Verification items for the finished model (mm, model axes). A direction names the side the tool comes from. Coordinates: 2 decimals unless noted, no trailing zeros. Order: outer loops, then holes, each group sorted by start corner. A loop starts at its lowest first (then second) coordinate and runs counter-clockwise, first axis right, second up. Notation, with made-up numbers: M 55.5,45 L 87.5,45 A28 cw 87.5,75 Z; hole C 50,45.25 d2. An arc over 180 degrees is marked long. Return JSON: item names as keys, results as strings. Group by question number.
1. Section check D-D, the plane z = -8. Record the cut outline in (x, y).
2. Set-up check for faces 1 (the flat face through (12, 1, 10)), 2 (the cylindrical face through (15.99, 1.12, 6.58)), 3 (the flat face through (12, 11, 10)), 4 (the flat face through (-12, 6, 0)): record each of +Z, -Z, +X, -X, +Y, -Y from which the full face is reachable in a straight line by a thin tool's end or side.
3. Section check A-A, the plane z = 9.5. Record the cut outline in (x, y).
4. Section check B-B, the plane y = 2. Record the cut outline in (x, z).
5. Material ranges on line 1 along X through (y, z) = (10.25, -2.25); line 2 along X through (y, z) = (5, 8.5); line 3 along Y through (x, z) = (12, 5.25), recorded low to high.
6. Section check C-C, the plane z = 4.75. Record the cut outline in (x, y), plus the area to 3 significant figures.
```python
from build123d import *

# Parameters (mm, degrees)
SCHIZZO1_W                   = 24
SCHIZZO1_H                   = 23
CORPOCENTRALE_DEPTH          = 12
SCHIZZO2_R                   = 6
ESTRUSIONE_ESTRUSIONE2_DEPTH = 3
SCHIZZO3_R                   = 5
ESTRUSIONE_ESTRUSIONE3_DEPTH = 2
SCHIZZO4_R                   = 2.5
ESTRUSIONE_ESTRUSIONE4_DEPTH = 3


with BuildPart() as part:
    # Schizzo1 → CorpoCentrale (new body)
    with BuildSketch(Plane(origin=(0, 0, 0), x_dir=(1, 0, 0), z_dir=(0, 1, 0))):
        Rectangle(SCHIZZO1_W, SCHIZZO1_H)
    extrude(amount=CORPOCENTRALE_DEPTH)

    # Schizzo2 → Estrusione-Estrusione2 (add)
    with BuildSketch(Plane(origin=(12, 0, 0), x_dir=(0, 0, -1), z_dir=(1, 0, 0))):
        with Locations(Location((-5.5, 6, 0), (0, 0, 180))):
            Circle(SCHIZZO2_R)
    extrude(amount=ESTRUSIONE_ESTRUSIONE2_DEPTH)

    # Schizzo3 → Estrusione-Estrusione3 (add)
    with BuildSketch(Plane(origin=(15, 0, 0), x_dir=(0, 0, -1), z_dir=(1, 0, 0))):
        with Locations((-5.5, 6)):
            Circle(SCHIZZO3_R)
    extrude(amount=ESTRUSIONE_ESTRUSIONE3_DEPTH)

    # Schizzo4 → Estrusione-Estrusione4 (add)
    with BuildSketch(Plane(origin=(17, 0, 0), x_dir=(0, 0, -1), z_dir=(1, 0, 0))):
        with Locations((-5.5, 6)):
            Circle(SCHIZZO4_R)
    extrude(amount=ESTRUSIONE_ESTRUSIONE4_DEPTH)


solid = part.part
```
Answers follow:
{
 "1": {"outline": "M -12,0 L 12,0 L 12,12 L -12,12 Z"},
 "2": {"face 1": "+Z, +X, -Y", "face 2": "+X", "face 3": "+Z, +X, +Y", "face 4": "+Z, -Z, -X, +Y, -Y"},
 "3": {"outline": "M -12,0 L 12,0 L 12,1.53 L 15,1.53 L 15,3 L 17,3 L 17,9 L 15,9 L 15,10.47 L 12,10.47 L 12,12 L -12,12 Z"},
 "4": {"outline": "M -12,-11.5 L 12,-11.5 L 12,1.03 L 15,1.03 L 15,2.5 L 17,2.5 L 17,8.5 L 15,8.5 L 15,9.97 L 12,9.97 L 12,11.5 L -12,11.5 Z"},
 "5": {"line 1": "-12 to 12", "line 2": "-12 to 17", "line 3": "0.01 to 11.99"},
 "6": {"outline": "M -12,0 L 12,0 L 12,0.05 L 15,0.05 L 15,1.06 L 17,1.06 L 17,3.62 L 20,3.62 L 20,8.38 L 17,8.38 L 17,10.94 L 15,10.94 L 15,11.95 L 12,11.95 L 12,12 L -12,12 Z", "area": "358 mm^2"}
}
